Autodesk Inventor part; units mm, degrees
ref_plane "YZ Plane" through (0, 0, 0) normal (1, 0, 0) x (0, 1, 0)
ref_plane "XZ Plane" through (0, 0, 0) normal (0, 1, 0) x (-1, 0, 0)
ref_plane "XY Plane" through (0, 0, 0) normal (0, 0, 1) x (1, 0, 0)
sketch "Sketch1" plane through (0, 0, 0) normal (0, 1, 0) x (-1, 0, 0)
  circle A0 centre (0, 0) radius 6.4135 construction
  line L0 (-3.2067, 5.5543) -> (3.2068, 5.5543)
  line L1 (-3.2067, 5.5543) -> (-6.4135, 0)
  line L2 (-6.4135, 0) -> (-3.2068, -5.5543)
  line L3 (-3.2068, -5.5543) -> (3.2067, -5.5543)
  line L4 (3.2067, -5.5543) -> (6.4135, 0)
  line L5 (6.4135, 0) -> (3.2068, 5.5543)
  circle A1 centre (0, 0) radius 4.0386
  dimension "d0" = 12.827
  dimension "d1" = 8.0772
extrude "Extrusion1" add sketch "Sketch1" along normal blind 6.4008
properties part number "denso-gates-15 spacer"
For this review, take the finished solid that the model builds, in its own axes (mm). Round coordinates to 2 decimals unless told otherwise and drop trailing zeros. Write each loop counter-clockwise with the first axis right and the second up, starting at its lowest first coordinate (ties: lowest second). Pieces come first, ordered by that corner, then holes. Notation, with made-up numbers: M 70,-34 L 119,-34 A21 cw 119,5 Z; hole C -31.75,-15.5 d3. An arc over 180 degrees is marked long. Write item = value, one per line. Start each with the question number.
(1) Clearance check with a flat-ended pin moving along its axis: pin 1 Ø3 at (y, z) = (5, -3) entering from +X. State where the tip first meets the part, or that it passes through.
(2) We need section D-D (x = 5.75). Give the boundary of the cut face in (y, z).
(3) The part is to be moulded in two halves that separate along X. For faces 1 (the face through (-4.788, 3.156, -2.816)), 2 (the face through (-3.852, 3.156, -1.213)), 3 (the face through (-4.2, 0, 0.1)), say which applies: +X half, -X half, draft (parallel to the pull), parting line (faces both ways), or undercut.
(4) We need section B-B (z = -2.5). Give the boundary of the cut face in (x, y), then the cut area to 3 significant figures.
(5) For line 1 along Z through (x, y) = (0, 4); line 2 along X through (y, z) = (3, 0.5); line 3 along Z through (x, y) = (-2.25, 4.75), list the stretches that pass through material, from the lowest coordinate up.
(6) We need section C-C (y = 1.5). Give the boundary of the cut face in (x, z), then the cut area to 3 significant figures.
(7) We need section A-A (x = 0). Give the boundary of the cut face in (y, z), then the cut area to 3 significant figures.
Results found:
q1.pin_1 = 5.55
q2.outline = M 0,-1.15 L 6.4,-1.15 L 6.4,1.15 L 0,1.15 Z
q3.face_1 = -X half
q3.face_2 = undercut
q3.face_3 = draft
q4.outline = M -4.97,0 L -3.17,0 L -3.17,6.4 L -4.97,6.4 Z; M 3.17,0 L 4.97,0 L 4.97,6.4 L 3.17,6.4 Z
q4.area = 23.0 mm²
q5.line_1 = -5.55 to -4.04, 4.04 to 5.55
q5.line_2 = -6.12 to -4.01, 4.01 to 6.12
q5.line_3 = -5.55 to -3.35, 3.35 to 5.55
q6.outline = M -6.41,0 L -3.21,-5.55 L 3.21,-5.55 L 6.41,0 L 3.21,5.55 L -3.21,5.55 Z; hole C 0,0 d8.08
q6.area = 55.6 mm²
q7.outline = M 0,-5.55 L 6.4,-5.55 L 6.4,-4.04 L 0,-4.04 Z; M 0,4.04 L 6.4,4.04 L 6.4,5.55 L 0,5.55 Z
q7.area = 19.4 mm²
